Check sheet for the modelled part. Datum: model origin and axes. Units: mm. A direction names the side the tool comes from. Round coordinates to 2 decimals unless told otherwise and drop trailing zeros. Loops run counter-clockwise (first coordinate to the right, second up) from the corner with the lowest first, then second, coordinate; pieces in that order, holes last. Notation, with made-up numbers: (-28, -1) - (8, -1) arc R32 cw to (8, 31) - close; hole circle Ø6 at (78.5, 60). An arc over 180 degrees is marked (long way). Return JSON: item names as keys, results as strings.
from build123d import *

# Parameters (mm, degrees)
SKETCH1_R           = 2
BOSS_EXTRUDE1_DEPTH = 6


with BuildPart() as part:
    # Sketch1 → Boss-Extrude1 (new body)
    with BuildSketch(Plane.XY):
        with BuildLine():
            Line((-10, 40.127930694), (-10, 0.127930694))
            Line((-10, 0.127930694), (-14.000572229, -17.872875451))
            ThreePointArc((-14.000572229, -17.872875451), (-10.109933276, -23.981807176), (-4, -20.092741267))
            Line((-4, -20.092741267), (0, -2.0945099))
            Line((0, -2.0945099), (-4, 2.9054901))
            Line((-4, 2.9054901), (0, 7.9054901))
            Line((0, 7.9054901), (-4, 12.9054901))
            Line((-4, 12.9054901), (0, 17.9054901))
            Line((0, 17.9054901), (-4, 22.9054901))
            Line((-4, 22.9054901), (0, 27.9054901))
            Line((0, 27.9054901), (-4, 32.9054901))
            Line((-4, 32.9054901), (0, 36.1054901))
            Line((0, 36.1054901), (0, 40.127930694))
            Line((0, 40.127930694), (-10, 40.127930694))
        make_face()
        with Locations((-5, -0.983289603)):
            Circle(SKETCH1_R, mode=Mode.SUBTRACT)
        with Locations((-9.000000331, -18.981520896)):
            Circle(SKETCH1_R, mode=Mode.SUBTRACT)
    extrude(amount=BOSS_EXTRUDE1_DEPTH)


solid = part.part
Q1. Scan lines: probe 1 along Y at (x, z) = (-9, 4.1); probe 2 along Y at (x, z) = (-5, 4.35); probe 3 along X at (y, z) = (31, 5.4). Record each from-to range of solid material in increasing order. Write a range as [from, to].
Answer key:
{"probe 1": "y = [-24.1, -20.98], [-16.98, 40.13]", "probe 2": "y = [-22.18, -2.98], [1.02, 40.13]", "probe 3": "x = [-10, -2.48]"}
Q2. Draft check along X on faces 4 (the face through (-7, -1, 3)), 5 (the face through (-10.22, -23.956, 2.958)), 6 (the face through (-2.03, 15.37, 2.96)). Enter one of: released by +X, released by -X, zero draft, split by the parting line, or undercut.
Answer key:
{"face 4": "undercut", "face 5": "split by the parting line", "face 6": "released by +X"}
Q3. Tool access check on faces 1 (the face through (-10, 20, 3)), 2 (the face through (0, 38, 3)), 3 (the face through (-2.03, 34.48, 2.96)). Record the directions out of +Z, -Z, +X, -X, +Y, -Y that give a thin tool (end or side, any length) a straight path to the whole face; none if there is none.
Answer key:
{"face 1": "+Z, -Z, -X, +Y", "face 2": "+Z, -Z, +X, +Y, -Y", "face 3": "+Z, -Z, +X"}
Q4. Sectioned sample at C-C (x = -5). Enter the section's corners in (y, z), plus the area to 3 significant figures.
Answer key:
{"outline": "(-22.18, 0) - (-2.98, 0) - (-2.98, 6) - (-22.18, 6) - close; (1.02, 0) - (40.13, 0) - (40.13, 6) - (1.02, 6) - close", "area": "350 mm²"}
Q5. Sectioned sample at D-D (y = 10). Enter the section's corners in (x, z).
Answer key:
{"outline": "(-10, 0) - (-1.68, 0) - (-1.68, 6) - (-10, 6) - close"}
Q6. Depth check by flat-ended pin: P1, Ø3, axis at x = -5, y = -0.98, coming from the +Z side; P2, Ø3, axis at y = 21, z = 3, coming from the -X side; P3, Ø1.5, axis at y = 32.5, z = 5, coming from the +X side. Enter the tip coordinate at first touch or a pass-through.
Answer key:
{"P1": "passes through", "P2": "stops at x = -10", "P3": "stops at x = -3.08"}
Q7. Sectioned sample at A-A (x = -9). Enter the section's corners in (y, z), plus the area to 3 significant figures.
Answer key:
{"outline": "(-24.1, 0) - (-20.98, 0) - (-20.98, 6) - (-24.1, 6) - close; (-16.98, 0) - (40.13, 0) - (40.13, 6) - (-16.98, 6) - close", "area": "361 mm²"}
Q8. Sectioned sample at B-B (z = 2.75). Enter the section's corners in (x, y).
Answer key:
{"outline": "(-14, -17.87) arc R5.12 ccw to (-4, -20.09) - (0, -2.09) - (-4, 2.91) - (0, 7.91) - (-4, 12.91) - (0, 17.91) - (-4, 22.91) - (0, 27.91) - (-4, 32.91) - (0, 36.11) - (0, 40.13) - (-10, 40.13) - (-10, 0.13) - close; hole circle Ø4 at (-9, -18.98); hole circle Ø4 at (-5, -0.98)"}
